```python
from build123d import *

# Parameters (mm, degrees)
SKETCH1_W           = 27.8
SKETCH1_H           = 28
SKETCH1_R           = 1
BOSS_EXTRUDE1_DEPTH = 1.3
SKETCH2_W           = 27
SKETCH2_H           = 19.5
BOSS_EXTRUDE2_DEPTH = 2


with BuildPart() as part:
    # Sketch1 → Boss-Extrude1 (new body)
    with BuildSketch(Plane.XY):
        with Locations((13.9, 14)):
            Rectangle(SKETCH1_W, SKETCH1_H)
        with Locations((25.8, 26)):
            Circle(SKETCH1_R, mode=Mode.SUBTRACT)
        with Locations((2, 26)):
            Circle(SKETCH1_R, mode=Mode.SUBTRACT)
        with Locations((25.8, 2)):
            Circle(SKETCH1_R, mode=Mode.SUBTRACT)
        with Locations((2, 2)):
            Circle(SKETCH1_R, mode=Mode.SUBTRACT)
    extrude(amount=BOSS_EXTRUDE1_DEPTH)

    # Sketch2 → Boss-Extrude2 (add)
    with BuildSketch(Plane.XY.offset(1.3)):
        with Locations((13.9, 13.85)):
            Rectangle(SKETCH2_W, SKETCH2_H)
    extrude(amount=BOSS_EXTRUDE2_DEPTH)


solid = part.part
```
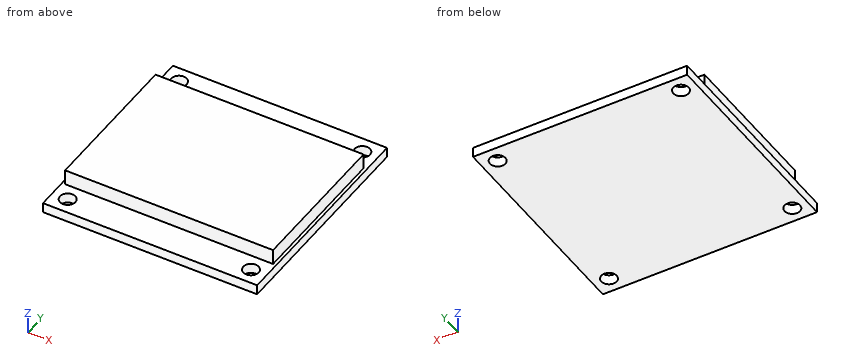
Input: part model. Units: mm. Frame: model coordinates. Round coordinates to 2 decimals unless told otherwise and drop trailing zeros. Loops run counter-clockwise (first coordinate to the right, second up) from the corner with the lowest first, then second, coordinate; pieces in that order, holes last. Notation, with made-up numbers: (-2, 28.5) -> (30, 28.5) arc R21 cw to (30, 41.5) -> close; hole circle Ø8 at (68, 29). An arc over 180 degrees is marked (long way). Write each question's results on one line, items separated by ' | '.
1. Section D-D (y = 15.25). Return loops of the section in (x, z), and give its area (3 significant figures).
Geometry results:
outline: (0, 0) -> (27.8, 0) -> (27.8, 1.3) -> (27.4, 1.3) -> (27.4, 3.3) -> (0.4, 3.3) -> (0.4, 1.3) -> (0, 1.3) -> close | area: 90.1 mm2
2. Ray query, line 1 (Y direction, x = 2, z = 0.7); line 2 (X direction, y = 17.5, z = 1.9); line 3 (Y direction, x = 2, z = 3.05). Return the intervals inside material, ascending. Write a range as from..to.
Geometry results:
line 1: 0..1, 3..25, 27..28 | line 2: 0.4..27.4 | line 3: 4.1..23.6
3. Section A-A (x = 25.8). Return loops of the section in (y, z).
Geometry results:
outline: (0, 0) -> (1, 0) -> (1, 1.3) -> (0, 1.3) -> close; (3, 0) -> (25, 0) -> (25, 1.3) -> (23.6, 1.3) -> (23.6, 3.3) -> (4.1, 3.3) -> (4.1, 1.3) -> (3, 1.3) -> close; (27, 0) -> (28, 0) -> (28, 1.3) -> (27, 1.3) -> close
4. Section B-B (y = 26). Return loops of the section in (x, z), and give its area (3 significant figures).
Geometry results:
outline: (0, 0) -> (1, 0) -> (1, 1.3) -> (0, 1.3) -> close; (3, 0) -> (24.8, 0) -> (24.8, 1.3) -> (3, 1.3) -> close; (26.8, 0) -> (27.8, 0) -> (27.8, 1.3) -> (26.8, 1.3) -> close | area: 30.9 mm2
5. Section C-C (x = 5.75). Return loops of the section in (y, z), and give its area (3 significant figures).
Geometry results:
outline: (0, 0) -> (28, 0) -> (28, 1.3) -> (23.6, 1.3) -> (23.6, 3.3) -> (4.1, 3.3) -> (4.1, 1.3) -> (0, 1.3) -> close | area: 75.4 mm2
6. First-contact query: P1, Ø1, axis at y = 10.5, z = 2.5, coming from the +X side; P2, Ø0.6, axis at x = 20, z = 2.5, coming from the -Y side. Flat tips, straight axial feed; report the tip coordinate or a pass-through.
Geometry results:
P1: x = 27.4 | P2: y = 4.1
